Autodesk Fusion 360 part; units mm, degrees
sketch "Sketch1" plane through (0, 0, 0) normal (0, 1, 0) x (1, 0, 0)
  line L0 (-50.5, -50) -> (4, -50)
  line L1 (4, -50) -> (4, 24.5)
  line L2 (4, 24.5) -> (-50.5, 24.5)
  line L3 (-50.5, 24.5) -> (-50.5, -50)
  dimension "d1" = 74.5
  dimension "d2" = 54.5
extrude "Extrude1" add sketch "Sketch1" along normal blind 50
shell "Shell1" thickness 2 removed faces 1 at (-14.1667, 0, 0.3333)
fillet "Fillet1" radius 5 1 edges at (-48.5, 24, -22.5)
fillet "Fillet2" radius 5 1 edges at (2, 24, -22.5)
fillet "Fillet3" radius 5 1 edges at (2, 24, 48)
fillet "Fillet4" radius 5 1 edges at (-48.5, 24, 48)
fillet "Fillet5" radius 5 8 edges at (-47.0355, 48, 46.5355) (-23.25, 48, 48) (0.5355, 48, 46.5355) (2, 48, 12.75) (0.5355, 48, -21.0355) (-23.25, 48, -22.5) (-47.0355, 48, -21.0355) (-48.5, 48, 12.75)
chamfer "Chamfer1" distance 2 angle 45 11 edges at (-50.5, 25, 50) (4, 25, 50) (4, 25, -24.5) (4, 50, 12.75) (4, 0, 12.75) (-23.25, 50, 50) (-23.25, 50, -24.5) (-50.5, 50, 12.75) (-50.5, 25, -24.5) (-23.25, 0, -24.5) (-23.25, 0, 50)
ref_plane "WorkPlane1" through (-23.25, 50, 12.75) normal (0, 1, 0) x (0, 0, 1)
sketch "Sketch2" plane through (0, 50, 0) normal (0, 1, 0) x (1, 0, 0)
  circle A0 centre (-22.9426, -23.5369) radius 4
  circle A1 centre (-22.9426, -23.5369) radius 3.5
  circle A2 centre (-32.9426, -9.5369) radius 1.5
  circle A3 centre (-12.9426, -9.5369) radius 1.5
  circle A4 centre (-12.9426, -27.5369) radius 1.5
  circle A5 centre (-32.9426, -27.5369) radius 1.5
extrude "Extrude2" add sketch "Sketch2" against normal blind 5 contours A2 | A3 | A4 | A5
extrude "Extrude3" cut sketch "Sketch2" against normal blind 7 contours A1
Geometry: final body of the model. Coordinates: model frame, mm. A direction names the side the tool comes from. Round coordinates to 2 decimals unless told otherwise and drop trailing zeros. Write each loop counter-clockwise with the first axis right and the second up, starting at its lowest first coordinate (ties: lowest second). Pieces come first, ordered by that corner, then holes. Notation, with made-up numbers: M 57,64.5 L 101,64.5 A24 ccw 101,94.5 Z; hole C 1,-13.5 d4. An arc over 180 degrees is marked long. Write item = value, one per line.
Item 1: Pin query (flat end, axial travel): P1, Ø1, axis at x = -39.5, z = 2, coming from the -Y side; P2, Ø2.5, axis at x = -13.5, z = 27, coming from the -Y side; P3, Ø4, axis at x = -22.94, z = 23.54, coming from the -Y side; P4, Ø3, axis at x = -43.5, z = 16, coming from the -Y side. Return the tip coordinate at first contact, or that it passes through.
Findings:
P1 = 48
P2 = 45
P3 = through
P4 = 47.77
Item 2: Access query for faces 1 (the face through (-33, 45, 28)), 2 (the face through (2.6, 1.2, 48.6)). Directions: +Z, -Z, +X, -X, +Y, -Y. A direction counts if a zero-diameter tool reaches every point of the face in a straight line with its end or side. Return the directions, or none.
Findings:
face_1 = -Y
face_2 = +Z, +X, -Y
Item 3: Material intervals for line 1 along X through (y, z) = (2.5, -6.5); line 2 along Z through (x, y) = (-7, 9); line 3 along Y through (x, z) = (-7.5, 41), sorted ascending. Write a range as [from, to].
Findings:
line_1 = [-50.5, -48.5], [2, 4]
line_2 = [-24.5, -22.5], [48, 50]
line_3 = [48, 50]
Item 4: Pull-direction query (X, two-part tool) for faces 3 (the face through (-23, 25, -24.5)), 4 (the face through (-24, 21, 48)), 5 (the face through (4, 25, 13)), 6 (the face through (-47.07, 21.8, 46.5)); classes: pulls with the +X half, pulls with the -X half, needs draft (parallel to the pull), parting line crosses it, or undercut.
Findings:
face_3 = needs draft
face_4 = undercut
face_5 = pulls with the +X half
face_6 = undercut
Item 5: Section query A-A on y = 9. Return loops of the section in (x, z), then the cut area to 3 significant figures.
Findings:
outline = M -50.5,-22.5 L -48.5,-24.5 L 2,-24.5 L 4,-22.5 L 4,48 L 2,50 L -48.5,50 L -50.5,48 Z; hole M -48.5,-17.5 A5 ccw -43.5,-22.5 L -3,-22.5 A5 ccw 2,-17.5 L 2,43 A5 ccw -3,48 L -43.5,48 A5 ccw -48.5,43 Z
area = 513 mm^2
